```python
from build123d import *

# Parameters (mm, degrees)
SKETCH1_R           = 1.35
BOSS_EXTRUDE2_DEPTH = 2
SKETCH3_R           = 1.35
BOSS_EXTRUDE3_DEPTH = 13
SKETCH5_R           = 1.35
BOSS_EXTRUDE4_DEPTH = 3
SKETCH6_W           = 6
SKETCH6_H           = 2.2
SKETCH6_W_2         = 2.1
SKETCH6_H_2         = 6
BOSS_EXTRUDE5_DEPTH = 4


with BuildPart() as part:
    # Sketch1 → Boss-Extrude2 (new body)
    with BuildSketch(Plane(origin=(0, 0, 0), x_dir=(1, 0, 0), z_dir=(0, 1, 0))):
        with BuildLine():
            Line((-15.5, 30), (-15.5, 11))
            Line((-15.5, 11), (-22.5, 11))
            ThreePointArc((-22.5, 11), (-25.5, 8), (-22.5, 5))
            Line((-22.5, 5), (-15.5, 5))
            Line((-15.5, 5), (-15.5, 0))
            Line((-15.5, 0), (16.5, 0))
            Line((16.5, 0), (16.5, 5))
            Line((16.5, 5), (23.5, 5))
            ThreePointArc((23.5, 5), (26.5, 8), (23.5, 11))
            Line((23.5, 11), (16.5, 11))
            Line((16.5, 11), (16.5, 30))
            Line((16.5, 30), (5, 30))
            Line((5, 30), (5, 34.5))
            ThreePointArc((5, 34.5), (0.5, 39), (-4, 34.5))
            Line((-4, 34.5), (-4, 30))
            Line((-4, 30), (-15.5, 30))
        make_face()
        with Locations(Location((-22.5, 8, 0), (0, 0, 270))):
            Circle(SKETCH1_R, mode=Mode.SUBTRACT)
        with Locations(Location((23.5, 8, 0), (0, 0, 270))):
            Circle(SKETCH1_R, mode=Mode.SUBTRACT)
    extrude(amount=BOSS_EXTRUDE2_DEPTH)

    # Sketch3 → Boss-Extrude3 (add)
    with BuildSketch(Plane(origin=(0, 2, 0), x_dir=(1, 0, 0), z_dir=(0, 1, 0))):
        with Locations(Location((0.5, 35, 0), (0, 0, 90))):
            Circle(SKETCH3_R)
    extrude(amount=BOSS_EXTRUDE3_DEPTH)

    # Sketch5 → Boss-Extrude4 (add)
    # profile 1 of 2: a face of its own
    with BuildSketch(Plane(origin=(0, 2, 0), x_dir=(1, 0, 0), z_dir=(0, 1, 0))):
        with BuildLine():
            Line((-15.5, 11), (-15.5, 5))
            Line((-15.5, 5), (-22.5, 5))
            ThreePointArc((-22.5, 5), (-25.5, 8), (-22.5, 11))
            Line((-22.5, 11), (-15.5, 11))
        make_face()
        with Locations(Location((-22.5, 8, 0), (0, 0, 270))):
            Circle(SKETCH5_R, mode=Mode.SUBTRACT)
    # profile 2 of 2: a face of its own
    with BuildSketch(Plane(origin=(0, 2, 0), x_dir=(1, 0, 0), z_dir=(0, 1, 0))):
        with BuildLine():
            Line((16.5, 11), (16.5, 5))
            Line((16.5, 5), (23.5, 5))
            ThreePointArc((23.5, 5), (26.5, 8), (23.5, 11))
            Line((23.5, 11), (16.5, 11))
        make_face()
        with Locations(Location((23.5, 8, 0), (0, 0, 270))):
            Circle(SKETCH5_R, mode=Mode.SUBTRACT)
    extrude(amount=BOSS_EXTRUDE4_DEPTH)

    # Sketch6 → Boss-Extrude5 (add)
    with BuildSketch(Plane(origin=(0, 0, 0), x_dir=(1, 0, 0), z_dir=(0, 1, 0))):
        with Locations((0.5, 1.1)):
            Rectangle(SKETCH6_W, SKETCH6_H)
        with Locations((-14.45, 16)):
            Rectangle(SKETCH6_W_2, SKETCH6_H_2)
        with Locations((15.45, 16)):
            Rectangle(SKETCH6_W_2, SKETCH6_H_2)
        with Locations((0.5, 31.3)):
            Rectangle(SKETCH6_W, SKETCH6_H)
    extrude(amount=BOSS_EXTRUDE5_DEPTH)


solid = part.part
```
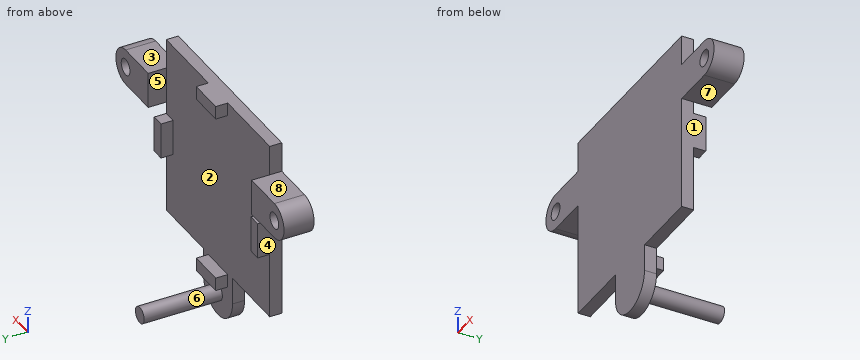
Model file for the job. Use its own axes, mm. Face numbers are marked on the shaded views. A direction names the side the tool comes from. Coordinates: 2 decimals unless noted, no trailing zeros. Write each loop counter-clockwise with the first axis right and the second up, starting at its lowest first coordinate (ties: lowest second). Pieces come first, ordered by that corner, then holes. Notation, with made-up numbers: (-22.5, 54) - (13.5, 54) arc R16 cw to (13.5, 63) - close; hole circle Ø7 at (72.5, -21.75). An arc over 180 degrees is marked (long way). One line per question, with ' | ' between items. Start each with the question number.
Q1. Pull direction X, two halves, no side cores. Call the marked faces 1, 2 and 3: pulls with the +X half, pulls with the -X half, needs draft (parallel to the pull), parting line crosses it, or undercut.
Q2. Pin check, flat tips, straight feed: pin 1 (1.5 mm diameter, centred on x = 17.5, z = -16.5, fed in from -Y); pin 2 (1 mm diameter, centred on y = 1, z = -3.5, fed in from +X); pin 3 (10 mm diameter, centred on x = 7.5, z = -15.5, fed in from -Y); pin 4 (1.6 mm diameter, centred on x = 1.5, y = 3, fed in from -Z). Stop position of each tip, or through.
Q3. Drill centre lines: line 1 (X direction, y = 3.5, z = -8); line 2 (X direction, y = 1.25, z = -8); line 3 (Y direction, x = -8, z = -9.5). Where is each one in solid material? Low to high. Write a range as [from, to].
Q4. Cut at C-C, the plane y = 13. List the corners of the cut face in (x, z), then the cut area to 3 significant figures.
Q5. Cut at A-A, the plane z = -8. List the corners of the cut face in (x, y).
Q6. 3-axis set-ups, long thin cutter, end or side, ignore diameter. For the marked faces 4, 5, 6, 7 and 8: which of +Z, -Z, +X, -X, +Y, -Y reach the whole face in a straight line?
Q7. Cut at B-B, the plane x = 0.5. List the corners of the cut face in (y, z), then the cut area to 3 significant figures.
Q8. Cut at D-D, the plane x = 10. List the corners of the cut face in (y, z), then the cut area to 3 significant figures.
Answer below:
1) face 1: pulls with the +X half | face 2: undercut | face 3: needs draft
2) pin 1: through | pin 2: x = 16.5 | pin 3: y = 0 | pin 4: z = -36.34
3) line 1: [-25.5, -23.85], [-21.15, -15.5], [16.5, 22.15], [24.85, 26.5] | line 2: [-25.5, -23.85], [-21.15, 22.15], [24.85, 26.5] | line 3: [0, 2]
4) outline: circle Ø2.7 at (0.5, -35) | area: 5.73 mm^2
5) outline: (-25.5, 0) - (-23.85, 0) - (-23.85, 5) - (-25.5, 5) - close; (-21.15, 0) - (22.15, 0) - (22.15, 5) - (16.5, 5) - (16.5, 2) - (-15.5, 2) - (-15.5, 5) - (-21.15, 5) - close; (24.85, 0) - (26.5, 0) - (26.5, 5) - (24.85, 5) - close
6) face 4: -Z, -X, +Y, -Y | face 5: +Z, +Y | face 6: +Y | face 7: -Z, +X, +Y, -Y | face 8: +Z, -X, +Y, -Y
7) outline: (0, -39) - (2, -39) - (2, -36.35) - (15, -36.35) - (15, -33.65) - (2, -33.65) - (2, -32.4) - (4, -32.4) - (4, -30.2) - (2, -30.2) - (2, -2.2) - (4, -2.2) - (4, 0) - (0, 0) - close | area: 122 mm^2
8) outline: (0, -30) - (2, -30) - (2, 0) - (0, 0) - close | area: 60.0 mm^2
